```python
from build123d import *

# Parameters (mm, degrees)
BOSS_EXTRUDE1_DEPTH = 2
SKETCH2_W           = 2
SKETCH2_H           = 7
BOSS_EXTRUDE2_DEPTH = 2.7
SKETCH3_R           = 0.4445
CUT_EXTRUDE1_DEPTH  = 10.052623929
SKETCH5_W           = 3.9
SKETCH5_H           = 4.7
BOSS_EXTRUDE3_DEPTH = 1
FILLET1_R           = 1
SKETCH6_R           = 0.4445
CUT_EXTRUDE2_DEPTH  = 9.100655838
FILLET2_R           = 1


with BuildPart() as part:
    # Sketch1 → Boss-Extrude1 (new body)
    with BuildSketch(Plane(origin=(0, 0, 0), x_dir=(1, 0, 0), z_dir=(0, 1, 0))):
        Polygon((2.075, -3.5), (2.825, -3.5), (3.825, -3.5), (4.825, -3.5), (4.825, 3.5), (3.825, 3.5), (2.825, 3.5), (2.075, 3.5), (-2.075, 3.5), (-4.075, 3.5), (-4.075, -3.5), (-2.075, -3.5), align=None)
    extrude(amount=BOSS_EXTRUDE1_DEPTH)

    # Sketch2 → Boss-Extrude2 (add)
    with BuildSketch(Plane(origin=(0, 2, 0), x_dir=(1, 0, 0), z_dir=(0, 1, 0))):
        with Locations((-3.075, 0)):
            Rectangle(SKETCH2_W, SKETCH2_H)
        with Locations((3.825, 0)):
            Rectangle(SKETCH2_W, SKETCH2_H)
    extrude(amount=BOSS_EXTRUDE2_DEPTH)

    # Sketch3 → Cut-Extrude1 (cut, through all)
    with BuildSketch(Plane.ZY.offset(-2.825)):
        with Locations((-1.25, 3.375)):
            Circle(SKETCH3_R)
        with Locations((2, 3.375)):
            Circle(SKETCH3_R)
    extrude(amount=-CUT_EXTRUDE1_DEPTH, mode=Mode.SUBTRACT)

    # Sketch5 → Boss-Extrude3 (add)
    with BuildSketch(Plane(origin=(0, 0, -3.5), x_dir=(-1, 0, 0), z_dir=(0, 0, -1))):
        with Locations((-2.875, 2.35)):
            Rectangle(SKETCH5_W, SKETCH5_H)
    extrude(amount=BOSS_EXTRUDE3_DEPTH)

    # Fillet1
    fillet1_edges = [part.edges().sort_by_distance(p)[0] for p in [
        (0.925, 1, -3.5),
    ]]
    fillet(fillet1_edges, radius=FILLET1_R - 0.0001)  # a hair under: the kernel refuses the full size

    # Sketch6 → Cut-Extrude2 (cut, through all)
    with BuildSketch(Plane.XZ):
        with Locations(Location((-0.575, 2, 0), (0, 0, 270))):
            Circle(SKETCH6_R)
        with Locations(Location((-0.575, -1.25, 0), (0, 0, 270))):
            Circle(SKETCH6_R)
    extrude(amount=-CUT_EXTRUDE2_DEPTH, mode=Mode.SUBTRACT)

    # Fillet2
    fillet2_edges = [part.edges().sort_by_distance(p)[0] for p in [
        (4.825, 0, -0.5),
        (-4.075, 0, 0),
    ]]
    fillet(fillet2_edges, radius=FILLET2_R)


solid = part.part
```
Geometry check sheet. Reference: the model listing, model coordinates, mm. A direction names the side the tool comes from. Give positions to 0.01 mm unless a question says otherwise; leave off trailing zeros. Order: outer loops, then holes, each group sorted by start corner. A loop starts at its lowest first (then second) coordinate and runs counter-clockwise, first axis right, second up. Notation, with made-up numbers: (80, -7.5) -> (119, -7.5) arc R15 ccw to (119, 17.5) -> close; hole circle Ø2 at (-38, -33.5). An arc over 180 degrees is marked (long way). Write each question's results on one line, items separated by ' | '. Start each with the question number.
(1) Mould release check, pull along Z, two halves, no side actions. Record for faces 1 (the face through (3, 2, -4.5)), 2 (the face through (-0.75, 0.99, 1.59)), 3 (the face through (4.825, 3, 0)): pulls with the +Z half, pulls with the -Z half, needs draft (parallel to the pull), parting line crosses it, or undercut.
(2) Sectioned sample at B-B (z = -3.25). Enter the section's corners in (x, y) (3 decimals), plus the area to 3 significant figures.
(3) Sectioned sample at C-C (y = 0.4). Give the number of separate pieces and of enclosed holes in the cut face, plus the area to 3 significant figures.
(4) Sectioned sample at D-D (x = -1.5). Enter the section's corners in (y, z), plus the area to 3 significant figures.
(5) Scan lines: line 1 (X direction, y = 1.1, z = -1.25) (1 decimal); line 2 (X direction, y = 4.35, z = 1.75) (3 decimals); line 3 (Y direction, x = 3.4, z = -1.25). Record each from-to range of solid material in increasing order.
(6) Gauge pin test, flat ends, axial feed: P1, Ø3, axis at x = 0.5, z = -0.5, coming from the +Y side; P2, Ø2, axis at x = 1.5, y = 3.5, coming from the +Z side. Record the tip position at first contact, or that the pin passes through.
(7) Access from +Z, -Z, +X, -X, +Y, -Y to the whole of each face (thin tool, end or side, straight path). Record for faces 4 (the face through (0.925, 3, -4)), 5 (the face through (2, 3, -3.5)), 6 (the face through (3.811, 2.981, -1.045)).
(8) Sectioned sample at A-A (z = -1.25). Enter the section's corners in (x, y) (1 decimal), plus the area to 3 significant figures.
Answer below:
1) face 1: pulls with the -Z half | face 2: undercut | face 3: needs draft
2) outline: (-4.075, 1) arc R1 ccw to (-3.075, 0) -> (3.825, 0) arc R1 ccw to (4.825, 1) -> (4.825, 4.7) -> (2.825, 4.7) -> (2.825, 2) -> (-2.075, 2) -> (-2.075, 4.7) -> (-4.075, 4.7) -> close | area: 28.2 mm2
3) separate pieces: 1 | enclosed holes: 2 | area: 62.2 mm2
4) outline: (0, -3.5) -> (2, -3.5) -> (2, 3.5) -> (0, 3.5) -> close | area: 14.0 mm2
5) line 1: -4.1 to -1, -0.1 to 4.8 | line 2: -4.075 to -2.075, 2.825 to 4.825 | line 3: 0 to 2.93, 3.82 to 4.7
6) P1: y = 2 | P2: z = -3.5
7) face 4: +Z, -Z, -X, +Y | face 5: +Z, +Y | face 6: +X
8) outline: (-4.1, 1) arc R1 ccw to (-3.1, 0) -> (-1, 0) -> (-1, 2) -> (-2.1, 2) -> (-2.1, 4.7) -> (-4.1, 4.7) -> close; (-0.1, 0) -> (3.8, 0) arc R1 ccw to (4.8, 1) -> (4.8, 2.9) -> (2.8, 2.9) -> (2.8, 2) -> (-0.1, 2) -> close; (2.8, 3.8) -> (4.8, 3.8) -> (4.8, 4.7) -> (2.8, 4.7) -> close | area: 24.6 mm2
